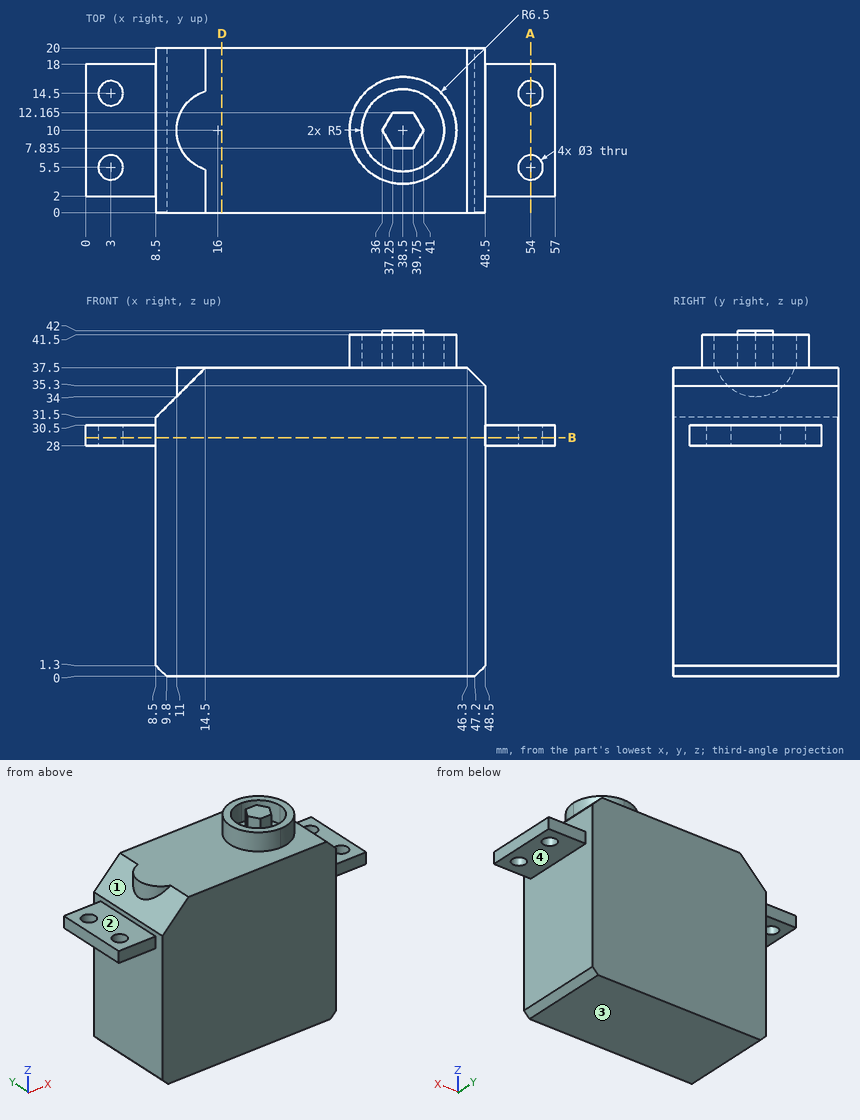
Job drawing, mm, ordinate dimensions from the low corner. One solid piece. A direction names the side the tool comes from. Round coordinates to 2 decimals unless told otherwise and drop trailing zeros. Write each loop counter-clockwise with the first axis right and the second up, starting at its lowest first coordinate (ties: lowest second). Pieces come first, ordered by that corner, then holes. Notation, with made-up numbers: (-9, 39) -> (-4, 39) arc R10 ccw to (-4, 48) -> close; hole circle Ø11 at (45, 19.25). An arc over 180 degrees is marked (long way). Answer as CSV lines item,"result".
1. Slice it at D-D, the plane x = 16.5. List the corners of the cut face in (y, z).
Resolved:
outline,"(0, 0) -> (20, 0) -> (20, 37.5) -> (0, 37.5) -> close"
2. Slice it at A-A, the plane x = 54. List the corners of the cut face in (y, z), plus the area to 3 significant figures.
Resolved:
outline,"(2, 28) -> (4, 28) -> (4, 30.5) -> (2, 30.5) -> close; (7, 28) -> (13, 28) -> (13, 30.5) -> (7, 30.5) -> close; (16, 28) -> (18, 28) -> (18, 30.5) -> (16, 30.5) -> close"
area,"25.0 mm²"
3. Tool access for the marked faces 1, 2, 3 and 4: list every direction of +Z, -Z, +X, -X, +Y, -Y with a clear straight run to the whole face (end or side of a thin tool).
Resolved:
face 1,"+Z, -X"
face 2,"+Z, -X, +Y, -Y"
face 3,"-Z, +X, -X, +Y, -Y"
face 4,"-Z, +X, +Y, -Y"
4. Slice it at B-B, the plane z = 29. List the corners of the cut face in (x, y).
Resolved:
outline,"(0, 2) -> (8.5, 2) -> (8.5, 0) -> (48.5, 0) -> (48.5, 2) -> (57, 2) -> (57, 18) -> (48.5, 18) -> (48.5, 20) -> (8.5, 20) -> (8.5, 18) -> (0, 18) -> close; hole circle Ø3 at (3, 5.5); hole circle Ø3 at (3, 14.5); hole circle Ø3 at (54, 5.5); hole circle Ø3 at (54, 14.5)"
5. Pin check, flat tips, straight feed: pin 1 Ø1.2 at (x, z) = (54, 29) entering from -Y; pin 2 Ø5 at (x, y) = (3, 5.5) entering from +Z; pin 3 Ø5 at (y, z) = (17, 5.5) entering from -X. Stop position of each tip, or through.
Resolved:
pin 1,"y = 2"
pin 2,"z = 30.5"
pin 3,"x = 8.5"
6. Drill centre lines: line 1 (Y direction, x = 3, z = 29); line 2 (Z direction, x = 6, y = 10.5); line 3 (Z direction, x = 30.5, y = 8). Where is each one in solid material? Low to high.
Resolved:
line 1,"2 to 4, 7 to 13, 16 to 18"
line 2,"28 to 30.5"
line 3,"0 to 37.5"
